from build123d import *

# Parameters (mm, degrees)
SKETCH2_R   = 3.175
SKETCH2_R_2 = 2.286


with BuildPart() as part:
    # Sweep1: sweep along a curve in space
    with BuildLine() as sweep1_path:
        Line((0, 0, 0), (31.75, 0, 0))
        ThreePointArc((31.75, 0, 0), (36.240128061, -1.859871939, 0), (38.1, -6.35, 0))
        Line((38.1, -6.35, 0), (38.1, -25.4, 0))
        ThreePointArc((38.1, -25.4, 0), (38.1, -29.890128061, 1.859871939), (38.1, -31.75, 6.35))
        Line((38.1, -31.75, 6.35), (38.1, -31.75, 6.999954124))
        ThreePointArc((38.1, -31.75, 6.999954124), (37.63596963, -31.75, 9.332792327), (36.314522938, -31.75, 11.310477062))
        Line((36.314522938, -31.75, 11.310477062), (33.609871939, -31.75, 14.015128061))
    # Sketch2 → Sweep1 (sweep)
    with BuildSketch(Plane(origin=(0, 0, 0), x_dir=(0, 0, -1), z_dir=(1, 0, 0))):
        Circle(SKETCH2_R)
        Circle(SKETCH2_R_2, mode=Mode.SUBTRACT)
    sweep(path=sweep1_path.line)


solid = part.part
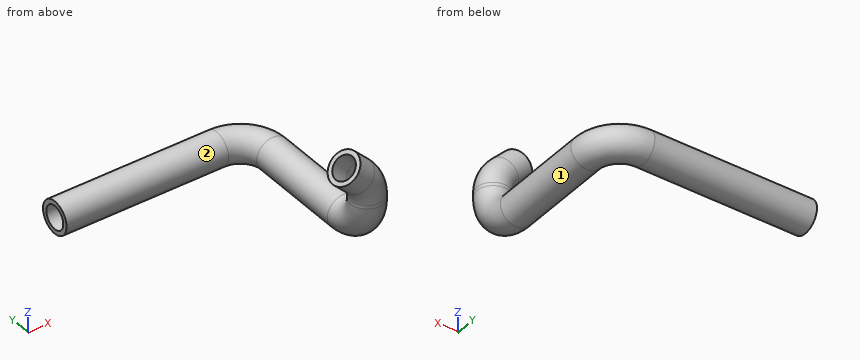
Design review of the part built by this model. Coordinates are the model's own, in mm. Face numbers are marked on the shaded views. A direction names the side the tool comes from. Give positions to 0.01 mm unless a question says otherwise; leave off trailing zeros. Loops run counter-clockwise (first coordinate to the right, second up) from the corner with the lowest first, then second, coordinate; pieces in that order, holes last. Notation, with made-up numbers: (4, 64.5) -> (21, 64.5) arc R37 cw to (21, 100.5) -> close; hole circle Ø8 at (42, 28). An arc over 180 degrees is marked (long way). One line per question, with ' | ' between items. Start each with the question number.
(1) For line 1 (Z direction, x = 38, y = -19); line 2 (Y direction, x = 24, z = 0) (3 decimals); line 3 (X direction, y = -31.75, z = 6.75) (3 decimals), list the stretches that pass through material, from the lowest coordinate up.
(2) We need section A-A (x = 8.5). State the section outline as (y, z) points (3 decimals).
(3) For the marked faces 1 and 2, list the 3-axis set-ups (+Z, -Z, +X, -X, +Y, -Y) from which the entire face can be reached by the end or side of a thin tool; tool diameter is ignored.
(4) We need section B-B (y = -8). State the section outline as (x, z) points (3 decimals).
(5) Insertion check: P1, Ø4, axis at y = -28.5, z = 7, coming from the +X side; P2, Ø8, axis at y = -14, z = -0.5, coming from the -X side (3 decimals); P3, Ø2.5, axis at x = 38.1, y = -31.75, coming from the -Z side. Each pin has a flat end and moves straight along its axis. Give the tip position at first contact, or say it passes through.
The answers:
1) line 1: z = -3.17 to -2.28, 2.28 to 3.17 | line 2: y = -3.175 to -2.286, 2.286 to 3.175 | line 3: x = 34.925 to 35.814, 40.386 to 41.275
2) outline: circle Ø6.35 at (0, 0); hole circle Ø4.572 at (0, 0)
3) face 1: none | face 2: -X
4) outline: circle Ø6.35 at (38.1, 0); hole circle Ø4.572 at (38.1, 0)
5) P1: stops at x = 41.02 | P2: stops at x = 34.925 | P3: stops at z = -1.69
